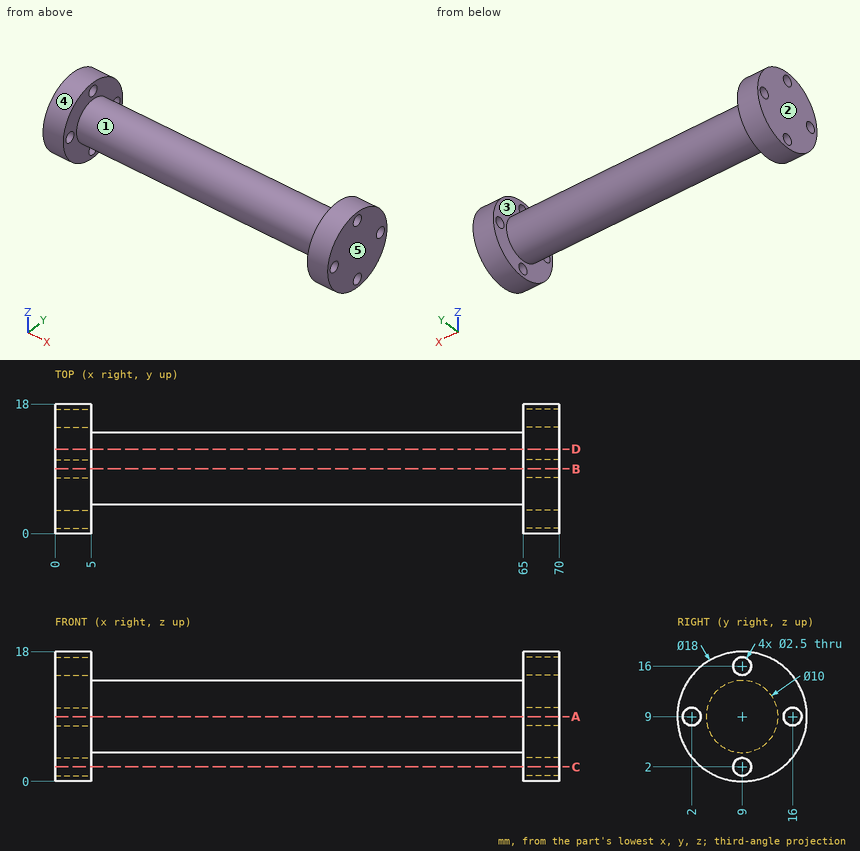
Verification items for this drawing (mm, ordinates from the low corner). A direction names the side the tool comes from. Round coordinates to 2 decimals unless told otherwise and drop trailing zeros. Order: outer loops, then holes, each group sorted by start corner. A loop starts at its lowest first (then second) coordinate and runs counter-clockwise, first axis right, second up. Notation, with made-up numbers: (17, -31.75) - (30, -31.75) arc R19 cw to (30, -24.75) - close; hole circle Ø2 at (-38, 6). An arc over 180 degrees is marked (long way). Answer as CSV lines item,"result". Start each with the question number.
1) Draft check along X on the marked faces 3, 4 and 5. Enter one of: +X half, -X half, draft (parallel to the pull), parting line (faces both ways), or undercut.
2) Section check D-D (y = 11.75). Record the cut outline in (x, z).
3) Tool access check on the marked faces 1 and 2. Record the directions out of +Z, -Z, +X, -X, +Y, -Y that give a thin tool (end or side, any length) a straight path to the whole face; none if there is none.
4) Section check C-C (z = 2). Record the cut outline in (x, y).
5) Section check A-A (z = 9). Record the cut outline in (x, y).
6) Scan lines: probe 1 along Y at (x, z) = (66.5, 9); probe 2 along X at (y, z) = (14.75, 6); probe 3 along Y at (x, z) = (24.5, 9). Record each from-to range of solid material in increasing order.
7) Depth check by flat-ended pin: pin 1 (8 mm diameter, centred on x = 50.5, y = 8.5, fed in from -Z); pin 2 (1.5 mm diameter, centred on x = 14, y = 12, fed in from -Z); pin 3 (4 mm diameter, centred on x = 23.5, y = 15, fed in from +Z). Enter the tip coordinate at first touch or a pass-through.
Determined:
1,face 3,"undercut"
1,face 4,"draft"
1,face 5,"+X half"
2,outline,"(0, 0.43) - (5, 0.43) - (5, 4.82) - (65, 4.82) - (65, 0.43) - (70, 0.43) - (70, 17.57) - (65, 17.57) - (65, 13.18) - (5, 13.18) - (5, 17.57) - (0, 17.57) - close"
3,face 1,"none"
3,face 2,"+Z, -Z, -X, +Y, -Y"
4,outline,"(0, 3.34) - (5, 3.34) - (5, 7.75) - (0, 7.75) - close; (0, 10.25) - (5, 10.25) - (5, 14.66) - (0, 14.66) - close; (65, 3.34) - (70, 3.34) - (70, 7.75) - (65, 7.75) - close; (65, 10.25) - (70, 10.25) - (70, 14.66) - (65, 14.66) - close"
5,outline,"(0, 0) - (5, 0) - (5, 0.75) - (0, 0.75) - close; (0, 3.25) - (5, 3.25) - (5, 4) - (65, 4) - (65, 3.25) - (70, 3.25) - (70, 14.75) - (65, 14.75) - (65, 14) - (5, 14) - (5, 14.75) - (0, 14.75) - close; (0, 17.25) - (5, 17.25) - (5, 18) - (0, 18) - close; (65, 0) - (70, 0) - (70, 0.75) - (65, 0.75) - close; (65, 17.25) - (70, 17.25) - (70, 18) - (65, 18) - close"
6,probe 1,"0 to 0.75, 3.25 to 14.75, 17.25 to 18"
6,probe 2,"0 to 5, 65 to 70"
6,probe 3,"4 to 14"
7,pin 1,"z = 4"
7,pin 2,"z = 4.53"
7,pin 3,"z = 12"
